```python
from build123d import *

# Parameters (mm, degrees)
ESBO_O1_R                = 470
RESSALTO_EXTRUS_O1_DEPTH = 6
ESBO_O2_R                = 275
CORTE_EXTRUS_O1_DEPTH    = 6
ESBO_O3_R                = 3
CORTE_EXTRUS_O2_DEPTH    = 6


with BuildPart() as part:
    # Esboço1 → Ressalto-extrusão1 (new body)
    with BuildSketch(Plane.XY):
        Circle(ESBO_O1_R)
    extrude(amount=RESSALTO_EXTRUS_O1_DEPTH)

    # Esboço2 → Corte-extrusão1 (cut)
    with BuildSketch(Plane.XY.offset(6)):
        Circle(ESBO_O2_R)
    extrude(amount=-CORTE_EXTRUS_O1_DEPTH, mode=Mode.SUBTRACT)

    # Esboço3 → Corte-extrusão2 (cut)
    with BuildSketch(Plane.XY.offset(6)):
        with Locations((0, -455)):
            Circle(ESBO_O3_R)
        with Locations((0, -288.71)):
            Circle(ESBO_O3_R)
    extrude(amount=-CORTE_EXTRUS_O2_DEPTH, mode=Mode.SUBTRACT)

    # Varredura1: sweep along a curve in space
    with BuildLine() as varredura1_path:
        ThreePointArc((470, 0, 0), (332.340187158, 332.340187158, 0), (0, 470, 0))
        ThreePointArc((0, 470, 0), (-332.340187158, 332.340187158, 0), (-470, 0, 0))
        ThreePointArc((-470, 0, 0), (-332.340187158, -332.340187158, 0), (0, -470, 0))
        ThreePointArc((0, -470, 0), (332.340187158, -332.340187158, 0), (470, 0, 0))
    # Esboço4 → Varredura1 (sweep)
    with BuildSketch(Plane(origin=(0, 0, 0), x_dir=(1, 0, 0), z_dir=(0, 1, 0))):
        with BuildLine():
            Line((-470, 0), (-470, 40))
            Line((-470, 40), (-540, 40))
            ThreePointArc((-540, 40), (-547.071067812, 37.071067812), (-550, 30))
            Line((-550, 30), (-550, -75))
            ThreePointArc((-550, -75), (-547.071067812, -82.071067812), (-540, -85))
            Line((-540, -85), (-470, -85))
            Line((-470, -85), (-470, 0))
        make_face()
    sweep(path=varredura1_path.line)


solid = part.part
```
Build history of the part. All positions in model axes, mm. A direction names the side the tool comes from. Round coordinates to 2 decimals unless told otherwise and drop trailing zeros. Order: outer loops, then holes, each group sorted by start corner. A loop starts at its lowest first (then second) coordinate and runs counter-clockwise, first axis right, second up. Notation, with made-up numbers: (87, -7.75) - (143, -7.75) arc R33 ccw to (143, 20.25) - close; hole circle Ø4 at (18.25, -27.75). An arc over 180 degrees is marked (long way). Use a Markdown table: item, result.
1) Pull direction X, two halves, no side cores. Call faces 1 (the face through (202, -202, 0)), 2 (the face through (262.3, 82.6, 3)), 3 (the face through (-198, -428, 85)): pulls with the +X half, pulls with the -X half, needs draft (parallel to the pull), parting line crosses it, or undercut.
Recorded:
| item | result |
|---|---|
| face 1 | undercut |
| face 2 | undercut |
| face 3 | needs draft |
2) Tool access for faces 4 (the face through (428, 198, -40)), 5 (the face through (202, -202, 6)): list every direction of +Z, -Z, +X, -X, +Y, -Y with a clear straight run to the whole face (end or side of a thin tool).
Recorded:
| item | result |
|---|---|
| face 4 | -Z, +X, -X, +Y, -Y |
| face 5 | +Z |
3) Flat gauge pins, fed straight in: pin 1 Ø8 at (x, y) = (0, -455) entering from +Z; pin 2 Ø4 at (y, z) = (270.5, 58) entering from -X; pin 3 Ø12 at (x, y) = (392.5, -251.5) entering from -Z; pin 4 Ø6 at (x, z) = (-264, -24.5) entering from +Y. Where does each tip first touch, or does it go through?
Recorded:
| item | result |
|---|---|
| pin 1 | stops at z = 6 |
| pin 2 | stops at x = -480.01 |
| pin 3 | stops at z = -40 |
| pin 4 | stops at y = 484.13 |
4) Wall check: L1, parallel to Y at x = 1.5, z = 13; L2, parallel to Y at x = 7.5, z = -1.5; L3, parallel to Z at x = 306.5, y = -75. Give the ranges that are in metal, low to high.
Recorded:
| item | result |
|---|---|
| L1 | y = -550 to -470, 470 to 550 |
| L2 | y = -549.95 to -469.94, 469.94 to 549.95 |
| L3 | z = 0 to 6 |
5) Saw through at A-A on z = 28.5. Write the cut outline in (x, y), and give its area (3 significant figures).
Recorded:
| item | result |
|---|---|
| outline | circle Ø1100 at (0, 0); hole circle Ø940 at (0, 0) |
| area | 256,000 mm² |
